from build123d import *

# Parameters (mm, degrees)
F0_W     = 60
F0_H     = 80
F1_DEPTH = 30
F2_W     = 56
F2_H     = 76
F3_DEPTH = 27.5
F4_SIZE  = 3
F5_SIZE  = 4.2
F6_SIZE2 = 1.7137776081
F6_SIZE  = 1.2


with BuildPart() as f1:
    # F0 (on Top) → F1 (new body)
    with BuildSketch(Plane.XY):
        with Locations((30, -40)):
            Rectangle(F0_W, F0_H)
    extrude(amount=F1_DEPTH)

    # F2 (on face) → F3 (cut, through all)
    with BuildSketch(Plane.XY.offset(30)):
        with Locations((30, -40)):
            Rectangle(F2_W, F2_H)
    extrude(amount=-F3_DEPTH, mode=Mode.SUBTRACT)

    # F4
    f4_edges = [f1.edges().sort_by_distance(p)[0] for p in [
        (58, -2, 16.25),
        (2, -2, 16.25),
        (58, -78, 16.25),
        (2, -78, 16.25),
    ]]
    chamfer(f4_edges, length=F4_SIZE)

    # F5
    f5_edges = [f1.edges().sort_by_distance(p)[0] for p in [
        (0, 0, 15),
        (60, 0, 15),
        (60, -80, 15),
        (0, -80, 15),
    ]]
    chamfer(f5_edges, length=F5_SIZE)

    # F6
    f6_edges = [f1.edges().sort_by_distance(p)[0] for p in [
        (30, 0, 0),
        (57.9, -2.1, 0),
        (2.1, -2.1, 0),
        (60, -40, 0),
        (0, -40, 0),
        (57.9, -77.9, 0),
        (2.1, -77.9, 0),
        (30, -80, 0),
    ]]
    f6_side = f1.faces().sort_by_distance((30, -40, 0))[0]
    chamfer(f6_edges, length=F6_SIZE, length2=F6_SIZE2, reference=f6_side)


solid = f1.part
Verification items for the finished model (mm, model axes). A direction names the side the tool comes from. Round coordinates to 2 decimals unless told otherwise and drop trailing zeros. Write each loop counter-clockwise with the first axis right and the second up, starting at its lowest first coordinate (ties: lowest second). Pieces come first, ordered by that corner, then holes.
(1) Section check A-A (x = 12). Enter the section's corners in (y, z), plus the area to 3 significant figures.
Returned:
outline: (-80, 1.71) - (-78.8, 0) - (-1.2, 0) - (0, 1.71) - (0, 30) - (-2, 30) - (-2, 2.5) - (-78, 2.5) - (-78, 30) - (-80, 30) - close
area: 308 mm2
(2) Material ranges on line 1 (Y direction, x = 51, z = 10.5); line 2 (X direction, y = -54.5, z = 12.5); line 3 (Z direction, x = 13, y = -32), recorded low to high.
Returned:
line 1: y = -80 to -78, -2 to 0
line 2: x = 0 to 2, 58 to 60
line 3: z = 0 to 2.5
(3) Depth check by flat-ended pin: pin 1 Ø5 at (x, y) = (28.5, -28) entering from +Z. Enter the tip coordinate at first touch or a pass-through.
Returned:
pin 1: stops at z = 2.5
(4) Mould release check, pull along Y, two halves, no side actions. Record for faces 3 (the flat face through (3, -4, 16)), 4 (the flat face through (2.1, -2.1, 15.7)), 5 (the flat face through (1, -37, 30)): pulls with the +Y half, pulls with the -Y half, needs draft (parallel to the pull), parting line crosses it, or undercut.
Returned:
face 3: undercut
face 4: pulls with the +Y half
face 5: needs draft
(5) Access from +Z, -Z, +X, -X, +Y, -Y to the whole of each face (thin tool, end or side, straight path). Record for faces 1 (the flat face through (2.489, -2.548, 0.869)), 2 (the flat face through (58, -40, 16)).
Returned:
face 1: -Z, -X, +Y
face 2: +Z
(6) Section check C-C (y = -31). Enter the section's corners in (x, z).
Returned:
outline: (0, 1.71) - (1.2, 0) - (58.8, 0) - (60, 1.71) - (60, 30) - (58, 30) - (58, 2.5) - (2, 2.5) - (2, 30) - (0, 30) - close
(7) Section check B-B (z = 11). Enter the section's corners in (x, y), plus the area to 3 significant figures.
Returned:
outline: (0, -75.8) - (4.2, -80) - (55.8, -80) - (60, -75.8) - (60, -4.2) - (55.8, 0) - (4.2, 0) - (0, -4.2) - close; hole (2, -75) - (5, -78) - (55, -78) - (58, -75) - (58, -5) - (55, -2) - (5, -2) - (2, -5) - close
area: 527 mm2
